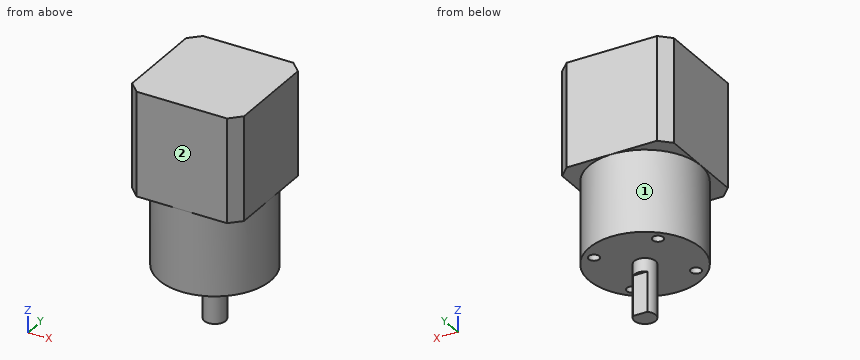
from build123d import *

# Parameters (mm, degrees)
SKETCH1_W           = 42
SKETCH1_H           = 42
BOSS_EXTRUDE1_DEPTH = 39
CHAMFER1_SIZE       = 4
SKETCH2_R           = 20.95
BOSS_EXTRUDE2_DEPTH = 30.6
SKETCH3_R           = 4
BOSS_EXTRUDE3_DEPTH = 20
CUT_EXTRUDE1_START  = -15
CUT_EXTRUDE1_DEPTH  = 15
SKETCH5_R           = 2
CUT_EXTRUDE2_DEPTH  = 20


with BuildPart() as part:
    # Sketch1 → Boss-Extrude1 (new body)
    with BuildSketch(Plane.XY):
        Rectangle(SKETCH1_W, SKETCH1_H)
    extrude(amount=BOSS_EXTRUDE1_DEPTH)

    # Chamfer1
    chamfer1_edges = [part.edges().sort_by_distance(p)[0] for p in [
        (21, -21, 19.5),
        (-21, -21, 19.5),
        (-21, 21, 19.5),
        (21, 21, 19.5),
    ]]
    chamfer(chamfer1_edges, length=CHAMFER1_SIZE)

    # Sketch2 → Boss-Extrude2 (add)
    with BuildSketch(Plane(origin=(0, 0, 0), x_dir=(-1, 0, 0), z_dir=(0, 0, -1))):
        Circle(SKETCH2_R)
    extrude(amount=BOSS_EXTRUDE2_DEPTH)

    # Sketch3 → Boss-Extrude3 (add)
    with BuildSketch(Plane(origin=(0, 0, -30.6), x_dir=(-1, 0, 0), z_dir=(0, 0, -1))):
        Circle(SKETCH3_R)
    extrude(amount=BOSS_EXTRUDE3_DEPTH)

    # Sketch4 → Cut-Extrude1 (cut)
    with BuildSketch(Plane(origin=(0, 0, -50.6), x_dir=(-1, 0, 0), z_dir=(0, 0, -1)).offset(CUT_EXTRUDE1_START)):
        with BuildLine():
            Line((-2.645751311, 3), (2.645751311, 3))
            ThreePointArc((2.645751311, 3), (0, 4), (-2.645751311, 3))
        make_face()
    extrude(amount=CUT_EXTRUDE1_DEPTH, mode=Mode.SUBTRACT)

    # Sketch5 → Cut-Extrude2 (cut)
    with BuildSketch(Plane(origin=(0, 0, -30.6), x_dir=(-1, 0, 0), z_dir=(0, 0, -1))):
        with Locations((12.02081528, 12.02081528)):
            Circle(SKETCH5_R)
        with Locations((12.02081528, -12.02081528)):
            Circle(SKETCH5_R)
        with Locations((-12.02081528, -12.02081528)):
            Circle(SKETCH5_R)
        with Locations((-12.02081528, 12.02081528)):
            Circle(SKETCH5_R)
    extrude(amount=-CUT_EXTRUDE2_DEPTH, mode=Mode.SUBTRACT)


solid = part.part
Can you work these out from the model? Positions are in its coordinate system, mm. Face numbers are marked on the shaded views. A direction names the side the tool comes from. Give positions to 0.01 mm unless a question says otherwise; leave off trailing zeros. Loops run counter-clockwise (first coordinate to the right, second up) from the corner with the lowest first, then second, coordinate; pieces in that order, holes last. Notation, with made-up numbers: M 48.5,33.25 L 53.5,33.25 A18 ccw 53.5,59.25 Z; hole C 78,47.25 d9. An arc over 180 degrees is marked long. One line per item, written item: value. Start each with the question number.
1) If we section it at D-D, the plane x = -18: Write out the boundary of the cut face in (y, z).
2) On a 3-axis mill with a long thin cutter (end or side, diameter ignored), from which of +Z, -Z, +X, -X, +Y, -Y can I reach the whole of each face in a straight line? I mean the marked faces 1 and 2. Say none if no direction works.
3) If we section it at B-B, the plane x = 0: Write out the boundary of the cut face in (y, z).
4) If we section it at C-C, the plane z = -22: Write out the boundary of the cut face in (x, y), and give its area (3 significant figures).
5) If I drill on line 1 (Z direction, x = -14.5, y = -18); line 2 (Z direction, x = 6, y = 1); line 3 (Y direction, x = 18, z = 3), over which ranges is the centre line in solid material (lowest first)? Write a range as [from, to].
6) I'm going to push flat-ended pins straight in: pin 1 (2 mm diameter, centred on x = -11.5, y = 11.5, fed in from -Z); pin 2 (0.8 mm diameter, centred on x = 1, y = 3.5, fed in from -Z); pin 3 (6 mm diameter, centred on x = 1, z = -40.5, fed in from +Y). Where does each tip first touch, or does it pass through?
7) If we section it at A-A, the plane y = 0: Write out the boundary of the cut face in (x, z), and give its area (3 significant figures).
Completed:
1. outline: M -20,0 L -10.72,0 L -10.72,-30.6 L 10.72,-30.6 L 10.72,0 L 20,0 L 20,39 L -20,39 Z
2. face 1: -Z
2. face 2: +Z, -Z, +X, -X, -Y
3. outline: M -21,0 L -20.95,0 L -20.95,-30.6 L -4,-30.6 L -4,-50.6 L 3,-50.6 L 3,-35.6 L 4,-35.6 L 4,-30.6 L 20.95,-30.6 L 20.95,0 L 21,0 L 21,39 L -21,39 Z
4. outline: C 0,0 d41.9; hole C -12.02,-12.02 d4; hole C -12.02,12.02 d4; hole C 12.02,-12.02 d4; hole C 12.02,12.02 d4
4. area: 1,330 mm^2
5. line 1: z = [0, 39]
5. line 2: z = [-30.6, 39]
5. line 3: y = [-20, 20]
6. pin 1: stops at z = -10.6
6. pin 2: stops at z = -35.6
6. pin 3: stops at y = 3
7. outline: M -21,0 L -20.95,0 L -20.95,-30.6 L -4,-30.6 L -4,-50.6 L 4,-50.6 L 4,-30.6 L 20.95,-30.6 L 20.95,0 L 21,0 L 21,39 L -21,39 Z
7. area: 3,080 mm^2
